```python
from build123d import *

# Parameters (mm, degrees)
FILLET2_R = 2


with BuildPart() as part:
    # Sketch2 → Revolve1 (revolve)
    with BuildSketch(Plane(origin=(0, 0, 0), x_dir=(0, 0, -1), z_dir=(1, 0, 0))):
        with BuildLine():
            Line((15.5224, 9.525), (9.5224, 9.525))
            Line((9.5224, 9.525), (9.5224, 15))
            Line((9.5224, 15), (7.9224, 15))
            Line((7.9224, 15), (7.9224, 13.45))
            Line((7.9224, 13.45), (6.5, 13.45))
            Line((6.5, 13.45), (6.5, 15))
            Line((6.5, 15), (-6.5, 15))
            Line((-6.5, 15), (-6.5, 20.55))
            Line((-6.5, 20.55), (-8.1, 20.55))
            Line((-8.1, 20.55), (-8.1, 17.85))
            Line((-8.1, 17.85), (-14.1, 17.85))
            Line((-14.1, 17.85), (-14.1, 16.35))
            Line((-14.1, 16.35), (-11.931122551, 16.35))
            ThreePointArc((-11.931122551, 16.35), (-9.543655274, 15.559361307), (-8.1, 13.5))
            Line((-8.1, 13.5), (2.5224, 13.5))
            ThreePointArc((2.5224, 13.5), (5.350827125, 12.328427125), (6.5224, 9.5))
            Line((6.5224, 9.5), (6.5224, 8.525))
            ThreePointArc((6.5224, 8.525), (7.108186438, 7.110786438), (8.5224, 6.525))
            Line((8.5224, 6.525), (15.5224, 6.525))
            Line((15.5224, 6.525), (15.5224, 9.525))
        make_face()
    revolve(axis=Axis((0, 0, 74.804360453), (0, 0, -1)))

    # Fillet2
    fillet2_edges = [part.edges().sort_by_distance(p)[0] for p in [
        (0, -9.525, -9.5224),
    ]]
    fillet(fillet2_edges, radius=FILLET2_R)


solid = part.part
```
CAD build for the part. Positions are in the model's coordinates, mm. A direction names the side the tool comes from. Give positions to 0.01 mm unless a question says otherwise; leave off trailing zeros. Order: outer loops, then holes, each group sorted by start corner. A loop starts at its lowest first (then second) coordinate and runs counter-clockwise, first axis right, second up. Notation, with made-up numbers: M 41.25,47.5 L 59.25,47.5 A26 cw 59.25,62.5 Z; hole C -20,46.5 d7. An arc over 180 degrees is marked long. Put each result on its own line as item: value. Start each with the question number.
(1) Saw through at A-A, the plane z = -4.25. Write the cut outline in (x, y), then the cut area to 3 significant figures.
(2) Drill centre lines: line 1 along X through (y, z) = (0, 0.25); line 2 along X through (y, z) = (-13.5, -6.25); line 3 along Z through (x, y) = (14, 11). Where is each one in solid material? Low to high.
(3) Saw through at B-B, the plane z = 5. Write the cut outline in (x, y), then the cut area to 3 significant figures.
(4) Mould opens along X. For faces 5 (the flat face through (4, -8, -6.522)), 6 (the flat face through (13.4, -3.4, -7.922)), 7 (the cylindrical face through (-5.796, -7.559, -13.494)) say: +X half, -X half, draft (parallel to the pull), parting line (faces both ways), or undercut.
(5) Which spindle directions (+Z, -Z, +X, -X, +Y, -Y) get a long thin tool onto all of the face, cutting with end or side? Do faces 1 (the flat face through (13.4, 3.4, -6.5)), 2 (the cylindrical face through (0.785, -17.833, 11.142)), 3 (the cylindrical face through (-20.061, -4.455, 7.311)), 4 (the flat face through (-11, -4, -9.522)). Say none if no direction does.
(6) Flat gauge pins, fed straight in: pin 1 Ø10 at (y, z) = (2.5, 5.5) entering from -X; pin 2 Ø1.5 at (x, y) = (13, 2.5) entering from +Z; pin 3 Ø24 at (x, y) = (5, 0) entering from -Z; pin 4 Ø8 at (x, z) = (8, -3.5) entering from -Y. Where does each tip first touch, or does it go through?
Check result:
1. outline: C 0,0 d30; hole C 0,0 d26.22
1. area: 167 mm2
2. line 1: x = -15 to -13.5, 13.5 to 15
2. line 2: x = -6.54 to 6.54
2. line 3: z = 6.5 to 14.1
3. outline: C 0,0 d30; hole C 0,0 d27
3. area: 134 mm2
4. face 5: undercut
4. face 6: draft
4. face 7: parting line
5. face 1: none
5. face 2: +Z
5. face 3: +Z, -Z
5. face 4: -Z
6. pin 1: stops at x = -20.55
6. pin 2: stops at z = 8.28
6. pin 3: stops at z = -15.52
6. pin 4: stops at y = -14.46
